```python
from build123d import *

# Parameters (mm, degrees)
F0_R     = 2
F1_DEPTH = 5
F2_DEPTH = 60
F4_DEPTH = 3
F5_R     = 4
F6_DEPTH = 8.001
F7_R     = 10


with BuildPart() as f1:
    # F0 (on Front) → F1 (new body)
    with BuildSketch(Plane.XZ):
        with BuildLine():
            Line((-20, 0), (-3, 0))
            Line((-3, 0), (-3, 20))
            Line((-3, 20), (0, 20))
            Line((0, 20), (3, 20))
            Line((3, 20), (3, 0))
            Line((3, 0), (20, 0))
            Line((20, 0), (30.1036297108, 17.5))
            ThreePointArc((30.1036297108, 17.5), (27.0675979174, 15.1703708686), (23.2735026919, 15.6698729811))
            Line((23.2735026919, 15.6698729811), (17.1132486541, 5))
            Line((17.1132486541, 5), (8, 5))
            Line((8, 5), (8, 20))
            Line((8, 20), (20.7735026919, 20))
            ThreePointArc((20.7735026919, 20), (22.237968786, 23.5355339059), (25.7735026919, 25))
            Line((25.7735026919, 25), (0, 25))
            Line((0, 25), (-25.7735026919, 25))
            ThreePointArc((-25.7735026919, 25), (-22.237968786, 23.5355339059), (-20.7735026919, 20))
            Line((-20.7735026919, 20), (-8, 20))
            Line((-8, 20), (-8, 5))
            Line((-8, 5), (-17.1132486541, 5))
            Line((-17.1132486541, 5), (-23.2735026919, 15.6698729811))
            ThreePointArc((-23.2735026919, 15.6698729811), (-27.0675979174, 15.1703708686), (-30.1036297108, 17.5))
            Line((-30.1036297108, 17.5), (-20, 0))
        make_face()
        with BuildLine():
            ThreePointArc((-25.7735026919, 25), (-30.1036297108, 22.5), (-30.1036297108, 17.5))
            ThreePointArc((-30.1036297108, 17.5), (-27.0675979174, 15.1703708686), (-23.2735026919, 15.6698729811))
            ThreePointArc((-23.2735026919, 15.6698729811), (-21.443375673, 17.5), (-20.7735026919, 20))
            ThreePointArc((-20.7735026919, 20), (-22.237968786, 23.5355339059), (-25.7735026919, 25))
        make_face()
        with Locations((-25.7735026919, 20)):
            Circle(F0_R, mode=Mode.SUBTRACT)
        with BuildLine():
            ThreePointArc((23.2735026919, 15.6698729811), (27.0675979174, 15.1703708686), (30.1036297108, 17.5))
            ThreePointArc((30.1036297108, 17.5), (30.6031318233, 18.7059047745), (30.7735026919, 20))
            ThreePointArc((30.7735026919, 20), (29.3090365978, 23.5355339059), (25.7735026919, 25))
            ThreePointArc((25.7735026919, 25), (22.237968786, 23.5355339059), (20.7735026919, 20))
            ThreePointArc((20.7735026919, 20), (21.443375673, 17.5), (23.2735026919, 15.6698729811))
        make_face()
        with Locations((25.7735026919, 20)):
            Circle(F0_R, mode=Mode.SUBTRACT)
    extrude(amount=F1_DEPTH)



with BuildPart() as f2:
    # F0 (on Front) → F2 (new body)
    with BuildSketch(Plane.XZ):
        Polygon((3, 0), (0, 0), (0, -8), (20, -8), (20, 0), align=None)
        Polygon((0, -8), (0, 0), (-3, 0), (-20, 0), (-20, -8), align=None)
    extrude(amount=F2_DEPTH)


with BuildPart() as f1_1:
    add(f1.part)

    add(f2.part)  # F4 merges F2
    # F3 (on Right) → F4 (join, symmetric)
    with BuildSketch(Plane.YZ):
        Polygon((0, 21.838214056), (-60, 0), (0, 0), align=None)
        Polygon((-31.6435909019, 5), (-10, 12.8776228509), (-10, 5), align=None, mode=Mode.SUBTRACT)
    extrude(amount=F4_DEPTH, both=True)

    # F5 (on Top) → F6 (cut, through all)
    with BuildSketch(Plane.XY):
        with Locations((-10, -50)):
            Circle(F5_R)
        with Locations((10, -50)):
            Circle(F5_R)
    extrude(amount=-F6_DEPTH, mode=Mode.SUBTRACT)

    # F7
    f7_edges = [f1_1.edges().sort_by_distance(p)[0] for p in [
        (-20, -60, -4),
        (20, -60, -4),
    ]]
    fillet(f7_edges, radius=F7_R)


solid = f1_1.part
```
For this review, take the finished solid that the model builds, in its own axes (mm). A direction names the side the tool comes from. Coordinates: 2 decimals unless noted, no trailing zeros. Loops run counter-clockwise (first coordinate to the right, second up) from the corner with the lowest first, then second, coordinate; pieces in that order, holes last. Notation, with made-up numbers: (-11.75, 74) - (39.25, 74) arc R9 cw to (39.25, 84) - close; hole circle Ø3 at (-10.5, -39). An arc over 180 degrees is marked (long way). Use one line per item in the form item = value. Start each with the question number.
1) For faces 1 (the face through (-14, -2, 20)), 2 (the face through (0, -30, -8)), 3 (the face through (12, -32, 0)), 4 (the face through (-11, -32, 0)), list the 3-axis set-ups (+Z, -Z, +X, -X, +Y, -Y) from which the entire face can be reached by the end or side of a thin tool; tool diameter is ignored.
2) For pin 1 (8 mm diameter, centred on y = -17, z = -4, fed in from -X); pin 2 (10 mm diameter, centred on y = -21.5, z = 9, fed in from +X); pin 3 (6 mm diameter, centred on x = 2, y = -6, fed in from +Z); pin 4 (5.5 mm diameter, centred on y = -3, z = 9, fed in from -X), all flat-tipped, find the tip position at first contact; note any pin that passes through.
3) Take a section at A-A (z = -2.5). State the section outline as (x, y) points.
4) Take a section at B-B (y = -18.5). State the section outline as (x, z) points.
5) Take a section at D-D (x = 0). State the section outline as (y, z) points, plus the area to 3 significant figures.
6) Draft analysis for pull direction X (two halves, no side actions). For faces 5 (the face through (-30.07, -2.46, 22.56)), 6 (the face through (0, -2, 25)), 7 (the face through (17.15, -56.99, -3.94)), 8 (the face through (8, -2, 12)), state which applies: released by +X, released by -X, zero draft, split by the parting line, or undercut.
7) To check wall thickness, follow probe 1 along X at (y, z) = (-51.5, -1.5); probe 2 along Y at (x, z) = (6, 20); probe 3 along Z at (x, y) = (-18.5, -24). State the ranges of each line that lie inside material, in increasing order. Write a range as from..to.
8) Take a section at C-C (x = 18). State the section outline as (y, z) points, plus the area to 3 significant figures.
From the geometry:
q1.face_1 = +Y, -Y
q1.face_2 = -Z, +X, -X, +Y, -Y
q1.face_3 = +Z, +X, -Y
q1.face_4 = +Z, -X, -Y
q2.pin_1 = -20
q2.pin_2 = 3
q2.pin_3 = 25
q2.pin_4 = -26.78
q3.outline = (-20, -50) arc R10 ccw to (-10, -60) - (10, -60) arc R10 ccw to (20, -50) - (20, 0) - (-20, 0) - close; hole circle Ø8 at (-10, -50); hole circle Ø8 at (10, -50)
q4.outline = (-20, -8) - (20, -8) - (20, 0) - (3, 0) - (3, 5) - (-3, 5) - (-3, 0) - (-20, 0) - close; (-3, 9.78) - (3, 9.78) - (3, 15.1) - (-3, 15.1) - close
q5.outline = (-60, -8) - (0, -8) - (0, 25) - (-5, 25) - (-5, 20.02) - (-60, 0) - close; hole (-31.64, 5) - (-10, 5) - (-10, 12.88) - close
q5.area = 1,070 mm2
q6.face_5 = released by -X
q6.face_6 = zero draft
q6.face_7 = released by +X
q6.face_8 = undercut
q7.probe_1 = -19.89..-13.71, -6.29..6.29, 13.71..19.89
q7.probe_2 = -5..0
q7.probe_3 = -8..0
q8.outline = (-56, -8) - (0, -8) - (0, 6.54) - (-5, 6.54) - (-5, 0) - (-56, 0) - close; (-5, 20) - (0, 20) - (0, 25) - (-5, 25) - close
q8.area = 506 mm2
